Geometry: final body of the model. Coordinates: model frame, mm. Face numbers are marked on the shaded views. Round coordinates to 2 decimals unless told otherwise and drop trailing zeros. Write each loop counter-clockwise with the first axis right and the second up, starting at its lowest first coordinate (ties: lowest second). Pieces come first, ordered by that corner, then holes. Notation, with made-up numbers: (8, 73.5) - (34, 73.5) arc R16 ccw to (34, 103.5) - close; hole circle Ø3 at (58.25, 47). An arc over 180 degrees is marked (long way). Write each question's results on one line, items separated by ' | '.
Autodesk Inventor part; units mm, degrees
ref_plane "YZ Plane" through (0, 0, 0) normal (1, 0, 0) x (0, 1, 0)
ref_plane "XZ Plane" through (0, 0, 0) normal (0, 1, 0) x (-1, 0, 0)
ref_plane "XY Plane" through (0, 0, 0) normal (0, 0, 1) x (1, 0, 0)
sketch "Sketch9" plane through (0, 0, -8.5889) normal (0, 0, 1) x (0.9992, 0.041, 0)
  circle A0 centre (0, 0) radius 27.1267
  circle A1 centre (0, 0) radius 20.1267
  circle A2 centre (-18.793, 7.2047) radius 1.5
  circle A3 centre (3.157, -19.8775) radius 1.5
  circle A4 centre (-7.3961, 16.9572) radius 3
  circle A5 centre (-7.3961, 16.9572) radius 3
  circle A6 centre (15.6359, 12.6728) radius 1.5
  dimension "d13" = 40.2533
  dimension "d14" = 54.2533
extrude "Extrusion1" add sketch "Sketch9" along normal blind 3 contours A0 | A1 A3 A2 A4 A6 | A6 A1 | A1 A6 | A3 A1 | A1 A3 | A4 A1 | A1 A4 | A2 A1 | A1 A2
sketch "Sketch2" plane through (0, 0, -5.5889) normal (0, 0, 1) x (1, 0, 0)
  circle A0 centre (0, 0) radius 16
  circle A1 centre (0, 0) radius 14
  dimension "d3" = 32
  dimension "d6" = 2
extrude "Extrusion3" add sketch "Sketch2" along normal blind 30
extrude "Extrusion4" cut sketch "Sketch2" against normal through all contours A1
extrude "Extrusion5" cut sketch "Sketch9" along normal through all contours A6 A1 | A1 A6 | A3 A1 | A1 A3 | A2 A1 | A1 A2
properties part number "SzenzorSzuportKerek" material "PPS Plastic"
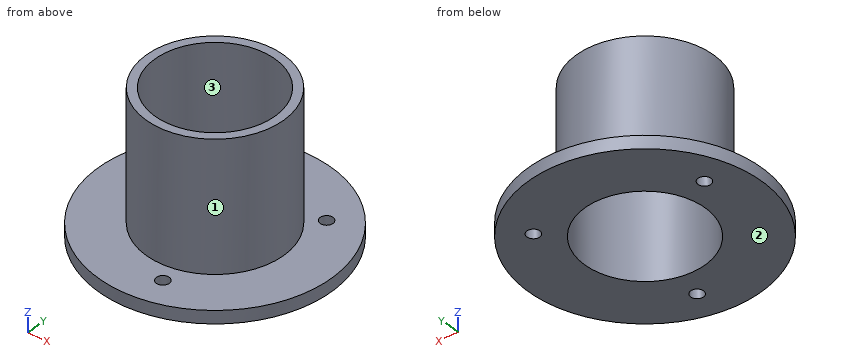
Q1. Ray query, line 1 along Y through (x, z) = (0, 14); line 2 along Z through (x, y) = (-8, 23); line 3 along X through (y, z) = (-11.5, 4). Return the intervals inside material, ascending.
Answer block:
line 1: -16 to -14, 14 to 16 | line 2: -8.59 to -5.59 | line 3: -11.12 to -7.98, 7.98 to 11.12
Q2. Section query C-C, the plane z = -2.5. Return loops of the section in (x, y).
Answer block:
outline: circle Ø32 at (0, 0); hole circle Ø28 at (0, 0)
Q3. Mould query, pull axis X, two halves, no side actions, for the marked faces 1, 2 and 3. Classes: pulls with the +X half, pulls with the -X half, needs draft (parallel to the pull), parting line crosses it, or undercut.
Answer block:
face 1: parting line crosses it | face 2: needs draft | face 3: undercut
Q4. Pin query (flat end, axial travel): pin 1 (4 mm diameter, centred on x = 14, z = 17, fed in from +Y); pin 2 (4 mm diameter, centred on x = 15.1, y = 13.3, fed in from +Z); pin 3 (4 mm diameter, centred on x = 1, z = 16.5, fed in from -Y). Return the tip coordinate at first contact, or that it passes through.
Answer block:
pin 1: y = 10.58 | pin 2: z = -5.59 | pin 3: y = -16
Q5. Section query A-A, the plane y = 0. Return loops of the section in (x, z).
Answer block:
outline: (-27.13, -8.59) - (-14, -8.59) - (-14, 24.41) - (-16, 24.41) - (-16, -5.59) - (-27.13, -5.59) - close; (14, -8.59) - (27.13, -8.59) - (27.13, -5.59) - (16, -5.59) - (16, 24.41) - (14, 24.41) - close
